Work out the finished part from the listing and answer in its coordinate system (mm). A direction names the side the tool comes from. Round coordinates to 2 decimals unless told otherwise and drop trailing zeros. Write each loop counter-clockwise with the first axis right and the second up, starting at its lowest first coordinate (ties: lowest second). Pieces come first, ordered by that corner, then holes.
from build123d import *

# Parameters (mm, degrees)
IZIM1_R                     = 1.5
Y_KSEKLIK_EKSTR_ZYON1_DEPTH = 3
KES_EKSTR_ZYON2_DEPTH       = 3


with BuildPart() as part:
    # Çizim1 → Yükseklik-Ekstrüzyon1 (new body)
    with BuildSketch(Plane.XY):
        with BuildLine():
            Line((-17.5, 100), (17.5, 100))
            Line((17.5, 100), (17.5, 75.773502692))
            ThreePointArc((17.5, 75.773502692), (18.839745962, 70.773502692), (22.5, 67.113248654))
            Line((22.5, 67.113248654), (46.871778265, 53.042195912))
            ThreePointArc((46.871778265, 53.042195912), (51.871778265, 51.70244995), (56.871778265, 53.042195912))
            Line((56.871778265, 53.042195912), (77.852540378, 65.155444566))
            Line((77.852540378, 65.155444566), (95.352540378, 34.844555434))
            Line((95.352540378, 34.844555434), (74.371778265, 22.73130678))
            ThreePointArc((74.371778265, 22.73130678), (70.711524227, 19.071052742), (69.371778265, 14.071052742))
            Line((69.371778265, 14.071052742), (69.371778265, -14.071052742))
            ThreePointArc((69.371778265, -14.071052742), (70.711524227, -19.071052742), (74.371778265, -22.73130678))
            Line((74.371778265, -22.73130678), (95.352540378, -34.844555434))
            Line((95.352540378, -34.844555434), (77.852540378, -65.155444566))
            Line((77.852540378, -65.155444566), (56.871778265, -53.042195912))
            ThreePointArc((56.871778265, -53.042195912), (51.871778265, -51.70244995), (46.871778265, -53.042195912))
            Line((46.871778265, -53.042195912), (22.5, -67.113248654))
            ThreePointArc((22.5, -67.113248654), (18.839745962, -70.773502692), (17.5, -75.773502692))
            Line((17.5, -75.773502692), (17.5, -100))
            Line((17.5, -100), (-17.5, -100))
            Line((-17.5, -100), (-17.5, -75.773502692))
            ThreePointArc((-17.5, -75.773502692), (-18.839745962, -70.773502692), (-22.5, -67.113248654))
            Line((-22.5, -67.113248654), (-46.871778265, -53.042195912))
            ThreePointArc((-46.871778265, -53.042195912), (-51.871778265, -51.70244995), (-56.871778265, -53.042195912))
            Line((-56.871778265, -53.042195912), (-77.852540379, -65.155444566))
            Line((-77.852540379, -65.155444566), (-95.352540379, -34.844555434))
            Line((-95.352540379, -34.844555434), (-74.371778265, -22.73130678))
            ThreePointArc((-74.371778265, -22.73130678), (-70.711524227, -19.071052742), (-69.371778265, -14.071052742))
            Line((-69.371778265, -14.071052742), (-69.371778265, 14.071052742))
            ThreePointArc((-69.371778265, 14.071052742), (-70.711524227, 19.071052742), (-74.371778265, 22.73130678))
            Line((-74.371778265, 22.73130678), (-95.352540378, 34.844555434))
            Line((-95.352540378, 34.844555434), (-77.852540378, 65.155444566))
            Line((-77.852540378, 65.155444566), (-56.871778265, 53.042195912))
            ThreePointArc((-56.871778265, 53.042195912), (-51.871778265, 51.70244995), (-46.871778265, 53.042195912))
            Line((-46.871778265, 53.042195912), (-22.5, 67.113248654))
            ThreePointArc((-22.5, 67.113248654), (-18.839745962, 70.773502692), (-17.5, 75.773502692))
            Line((-17.5, 75.773502692), (-17.5, 100))
        make_face()
        with Locations((-12.5, 95)):
            Circle(IZIM1_R, mode=Mode.SUBTRACT)
        with Locations((12.5, 95)):
            Circle(IZIM1_R, mode=Mode.SUBTRACT)
        with Locations((0, 75)):
            Circle(IZIM1_R, mode=Mode.SUBTRACT)
        with Locations((76.022413359, 58.325317547)):
            Circle(IZIM1_R, mode=Mode.SUBTRACT)
        with Locations((88.522413359, 36.674682453)):
            Circle(IZIM1_R, mode=Mode.SUBTRACT)
        with Locations((64.951905284, 37.5)):
            Circle(IZIM1_R, mode=Mode.SUBTRACT)
        with Locations((88.522413359, -36.674682453)):
            Circle(IZIM1_R, mode=Mode.SUBTRACT)
        with Locations((76.02241336, -58.325317547)):
            Circle(IZIM1_R, mode=Mode.SUBTRACT)
        with Locations((64.951905284, -37.5)):
            Circle(IZIM1_R, mode=Mode.SUBTRACT)
        with Locations((12.5, -95)):
            Circle(IZIM1_R, mode=Mode.SUBTRACT)
        with Locations((-12.5, -95)):
            Circle(IZIM1_R, mode=Mode.SUBTRACT)
        with Locations((0, -75)):
            Circle(IZIM1_R, mode=Mode.SUBTRACT)
        with Locations((-76.022413359, -58.325317547)):
            Circle(IZIM1_R, mode=Mode.SUBTRACT)
        with Locations((-88.522413359, -36.674682453)):
            Circle(IZIM1_R, mode=Mode.SUBTRACT)
        with Locations((-64.951905284, -37.5)):
            Circle(IZIM1_R, mode=Mode.SUBTRACT)
        with Locations((-88.522413359, 36.674682453)):
            Circle(IZIM1_R, mode=Mode.SUBTRACT)
        with Locations((-76.022413359, 58.325317547)):
            Circle(IZIM1_R, mode=Mode.SUBTRACT)
        with Locations((-64.951905284, 37.5)):
            Circle(IZIM1_R, mode=Mode.SUBTRACT)
    extrude(amount=Y_KSEKLIK_EKSTR_ZYON1_DEPTH)

    # Çizim2 → Kes-Ekstrüzyon2 (cut)
    with BuildSketch(Plane.XY.offset(3)):
        with BuildLine():
            Line((-17.5, 24.75), (17.5, 24.75))
            ThreePointArc((17.5, 24.75), (22.25, 20), (17.5, 15.25))
            Line((17.5, 15.25), (-17.5, 15.25))
            ThreePointArc((-17.5, 15.25), (-22.25, 20), (-17.5, 24.75))
        make_face()
        with BuildLine():
            Line((-20, -15.25), (20, -15.25))
            ThreePointArc((20, -15.25), (24.75, -20), (20, -24.75))
            Line((20, -24.75), (-20, -24.75))
            ThreePointArc((-20, -24.75), (-24.75, -20), (-20, -15.25))
        make_face()
    extrude(amount=-KES_EKSTR_ZYON2_DEPTH, mode=Mode.SUBTRACT)


solid = part.part
Q1. Find section D-D (y = -45.5). Determine the outline of the cut face in (x, z), plus the area to 3 significant figures.
Q2. The mould has two halves that part along X. Classify faces 5 (the face through (24.75, -19.9, 1.52)), 6 (the face through (-18.8, -70.84, 1.48)), 7 (the face through (85.009, 28.873, 1.479)): +X half, -X half, draft (parallel to the pull), parting line (faces both ways), or undercut.
Q3. A tool of negligible diameter and unlimited length cuts with its end or side. For faces 1 (the face through (-67.509, 59.184, 1.479)), 2 (the face through (34.856, -59.979, 1.479)), 3 (the face through (-70.675, 19.007, 1.479)), 4 (the face through (84.715, -28.703, 1.479)), from which of +Z, -Z, +X, -X, +Y, -Y can it reach the whole face along a straight path? Write none if from no direction.
Q4. Find section A-A (y = 20). Determine the outline of the cut face in (x, z).
Q5. Find section C-C (z = 1.55). Count the separate pieces of the cut face and the enclosed holes in it, plus the area to 3 significant figures.
Q6. Given pin 1 (2 mm diameter, centred on x = -36.5, y = 46, fed in from -Z); pin 2 (1 mm diameter, centred on y = 56, z = 0.5, fed in from +X), each flat-ended and moving along its own axis, determine where each tip first touches the part or whether it passes through.
Q7. Find the intervals of material crossed by L1, parallel to X at y = -95, z = 0.6; L2, parallel to Y at x = -2.5, z = 2.5; L3, parallel to Y at x = -12.5, z = 2.3, in increasing order.
Q8. Find section B-B (x = -72). Determine the outline of the cut face in (y, z).
Report:
1. outline: (-89.2, 0) - (89.2, 0) - (89.2, 3) - (-89.2, 3) - close
1. area: 535 mm2
2. face 5: undercut
2. face 6: -X half
2. face 7: +X half
3. face 1: +Z, -Z, +Y
3. face 2: +Z, -Z, -Y
3. face 3: +Z, -Z, -X
3. face 4: +Z, -Z, +X
4. outline: (-71.32, 0) - (-22.25, 0) - (-22.25, 3) - (-71.32, 3) - close; (22.25, 0) - (71.32, 0) - (71.32, 3) - (22.25, 3) - close
5. separate pieces: 1
5. enclosed holes: 20
5. area: 21,000 mm2
6. pin 1: stops at z = 0
6. pin 2: stops at x = 83.43
7. L1: x = -17.5 to -14, -11 to 11, 14 to 17.5
7. L2: y = -100 to -24.75, -15.25 to 15.25, 24.75 to 100
7. L3: y = -100 to -96.5, -93.5 to -24.75, -15.25 to 15.25, 24.75 to 93.5, 96.5 to 100
8. outline: (-61.78, 0) - (-20.83, 0) - (-20.83, 3) - (-61.78, 3) - close; (20.83, 0) - (61.78, 0) - (61.78, 3) - (20.83, 3) - close
